```python
from build123d import *

# Parameters (mm, degrees)
F0_W     = 18
F0_H     = 145
F1_DEPTH = 720
F2_W     = 100
F2_H     = 18
F3_DEPTH = 18.001
F5_DEPTH = 18


with BuildPart() as f1:
    # F0 (on Top) → F1 (new body)
    with BuildSketch(Plane.XY):
        with Locations((-9, 0)):
            Rectangle(F0_W, F0_H)
    extrude(amount=F1_DEPTH)

    # F2 (on face) → F3 (cut, through all)
    with BuildSketch(Plane.YZ):
        with Locations((0, 34)):
            Rectangle(F2_W, F2_H)
        with Locations((0, 252)):
            Rectangle(F2_W, F2_H)
        with Locations((0, 470)):
            Rectangle(F2_W, F2_H)
    extrude(amount=-F3_DEPTH, mode=Mode.SUBTRACT)

    # F4 (on face) → F5 (cut)
    with BuildSketch(Plane.XY.offset(720)):
        Polygon((-18, 0), (-18, -10), (0, -7.5), (0, 0), (0, 7.5), (-18, 10), align=None)
        Polygon((0, -18.5), (-18, -16), (-18, -36), (0, -33.5), align=None)
        Polygon((-18, 36), (-18, 16), (0, 18.5), (0, 33.5), align=None)
        Polygon((-18, 62), (-18, 42), (0, 44.5), (0, 59.5), align=None)
        Polygon((0, -44.5), (-18, -42), (-18, -62), (0, -59.5), align=None)
    extrude(amount=-F5_DEPTH, mode=Mode.SUBTRACT)


solid = f1.part
```
The listing builds one solid part. Answer for the finished solid, in the listing's coordinates (mm). A direction names the side the tool comes from. Round coordinates to 2 decimals unless told otherwise and drop trailing zeros. Loops run counter-clockwise (first coordinate to the right, second up) from the corner with the lowest first, then second, coordinate; pieces in that order, holes last. Notation, with made-up numbers: (70, 31.25) - (76, 31.25) arc R29 cw to (76, 56.25) - close; hole circle Ø6 at (50.5, 70.25). An arc over 180 degrees is marked (long way). Use one line per item in the form item = value. Start each with the question number.
1. For a pull along Z with two mould halves and no side action, classify faces 1 (the face through (-9, -26, 702)), 2 (the face through (-9, -1, 479)), 3 (the face through (-9.13, -60.77, 711.13)) as pulls with the +Z half, pulls with the -Z half, needs draft (parallel to the pull), parting line crosses it, or undercut.
2. Given pin 1 Ø9 at (x, y) = (-8.5, 8.5) entering from +Z; pin 2 Ø6 at (x, y) = (-14, -5) entering from +Z, each flat-ended and moving along its own axis, determine where each tip first touches the part or whether it passes through.
3. Consider line 1 (Z direction, x = -11.25, y = 28); line 2 (Z direction, x = -13, y = 39.5); line 3 (Z direction, x = -0.75, y = 56.5). Determine where each line is inside the solid, lowest interval first. Write a range as [from, to].
4. The part is cut by section B-B on x = -12.25. Give the number of separate pieces and of enclosed holes in the cut face, then the cut area to 3 significant figures.
5. A tool of negligible diameter and unlimited length cuts with its end or side. For faces 4 (the face through (-9, 72.5, 355)), 5 (the face through (-9, -1, 261)), 6 (the face through (-9.13, -8.77, 711.13)), from which of +Z, -Z, +X, -X, +Y, -Y can it reach the whole face along a straight path? Write none if from no direction.
6. The part is cut by section A-A on y = 26.5. Determine the outline of the cut face in (x, z).
Geometry check:
q1.face_1 = pulls with the +Z half
q1.face_2 = undercut
q1.face_3 = needs draft
q2.pin_1 = 720
q2.pin_2 = 702
q3.line_1 = [0, 25], [43, 243], [261, 461], [479, 702]
q3.line_2 = [0, 25], [43, 243], [261, 461], [479, 720]
q3.line_3 = [0, 702]
q4.separate_pieces = 1
q4.enclosed_holes = 3
q4.area = 97,300 mm^2
q5.face_4 = +Z, -Z, +X, -X, +Y
q5.face_5 = +X, -X
q5.face_6 = +Z, -X
q6.outline = (-18, 0) - (0, 0) - (0, 25) - (-18, 25) - close; (-18, 43) - (0, 43) - (0, 243) - (-18, 243) - close; (-18, 261) - (0, 261) - (0, 461) - (-18, 461) - close; (-18, 479) - (0, 479) - (0, 702) - (-18, 702) - close
